```python
from build123d import *

# Parameters (mm, degrees)
F0_W     = 152.4
F0_H     = 25.4
F1_DEPTH = 12.7
F2_DEPTH = 25.4
F3_R     = 5.08


with BuildPart() as f1:
    # F0 (on Front) → F1 (new body, symmetric)
    with BuildSketch(Plane.XZ):
        Rectangle(F0_W, F0_H)
    extrude(amount=F1_DEPTH, both=True)

    # F2 (add): a face of the model
    f2_faces = [f1.faces().sort_by_distance(p)[0] for p in [
        (0, -12.7, 0),
    ]]
    extrude(f2_faces, amount=F2_DEPTH)

    # F3
    f3_edges = [f1.edges().sort_by_distance(p)[0] for p in [
        (0, -38.1, 12.7),
        (0, -38.1, -12.7),
        (0, 12.7, 12.7),
        (0, 12.7, -12.7),
    ]]
    fillet(f3_edges, radius=F3_R)


solid = f1.part
```
Part model, mm, in its own coordinate system. Give positions to 0.01 mm unless a question says otherwise; leave off trailing zeros. Order: outer loops, then holes, each group sorted by start corner. A loop starts at its lowest first (then second) coordinate and runs counter-clockwise, first axis right, second up. Notation, with made-up numbers: (82, -32) - (101, -32) arc R19 ccw to (101, -8) - close; hole circle Ø9 at (-27, 12.25). An arc over 180 degrees is marked (long way). Use one line per item in the form item = value.
Item 1: Slice it at B-B on z = 11. Give the cut face in (x, y).
Solution:
outline = (-76.2, -36.81) - (76.2, -36.81) - (76.2, 11.41) - (-76.2, 11.41) - close
Item 2: Slice it at A-A on x = 51.5. Give the cut face in (y, z).
Solution:
outline = (-38.1, -7.62) arc R5.08 ccw to (-33.02, -12.7) - (7.62, -12.7) arc R5.08 ccw to (12.7, -7.62) - (12.7, 7.62) arc R5.08 ccw to (7.62, 12.7) - (-33.02, 12.7) arc R5.08 ccw to (-38.1, 7.62) - close
Item 3: Slice it at C-C on z = -9.75. Give the cut face in (x, y).
Solution:
outline = (-76.2, -37.63) - (76.2, -37.63) - (76.2, 12.23) - (-76.2, 12.23) - close
Item 4: Probe probe 1 along Y at (x, z) = (-35.5, 9.25); probe 2 along Y at (x, z) = (-51.5, 10.75); probe 3 along Z at (x, y) = (-16, -35). List the from-to ranges inside material, lowest first. Write a range as from..to.
Solution:
probe_1 = -37.83..12.43
probe_2 = -37.02..11.62
probe_3 = -12.3..12.3
